Geometry: see drawing. Coordinates: mm, zero at the bounding-box minimum. A direction names the side the tool comes from. Give positions to 0.01 mm unless a question says otherwise; leave off trailing zeros. Write each loop counter-clockwise with the first axis right and the second up, starting at its lowest first coordinate (ties: lowest second). Pieces come first, ordered by that corner, then holes. Notation, with made-up numbers: (61.25, 89) - (104.25, 89) arc R13 ccw to (104.25, 101) - close; hole circle Ø9 at (56, -31.5). An arc over 180 degrees is marked (long way). Use a Markdown table: item, result. Add a question column.
1. Set-up query: the marked faces 1 and 2. Return all of +Z, -Z, +X, -X, +Y, -Y with unobstructed straight access to the full face (end or side cutting, diameter ignored); none if empty.
2. Section query B-B, the plane x = 38.5. Return loops of the section in (y, z).
3. Material intervals for probe 1 along Y at (x, z) = (8.5, 40.5); probe 2 along X at (y, z) = (122.5, 32), sorted ascending.
4. Section query A-A, the plane z = 35. Return loops of the section in (x, y), plus the area to 3 significant figures.
5. Pin query (flat end, axial travel): pin 1 (7.5 mm diameter, centred on x = 35, z = 41.5, fed in from +Y); pin 2 (12 mm diameter, centred on x = 18, z = 12.5, fed in from -Y). Return the tip coordinate at first contact, or that it passes through.
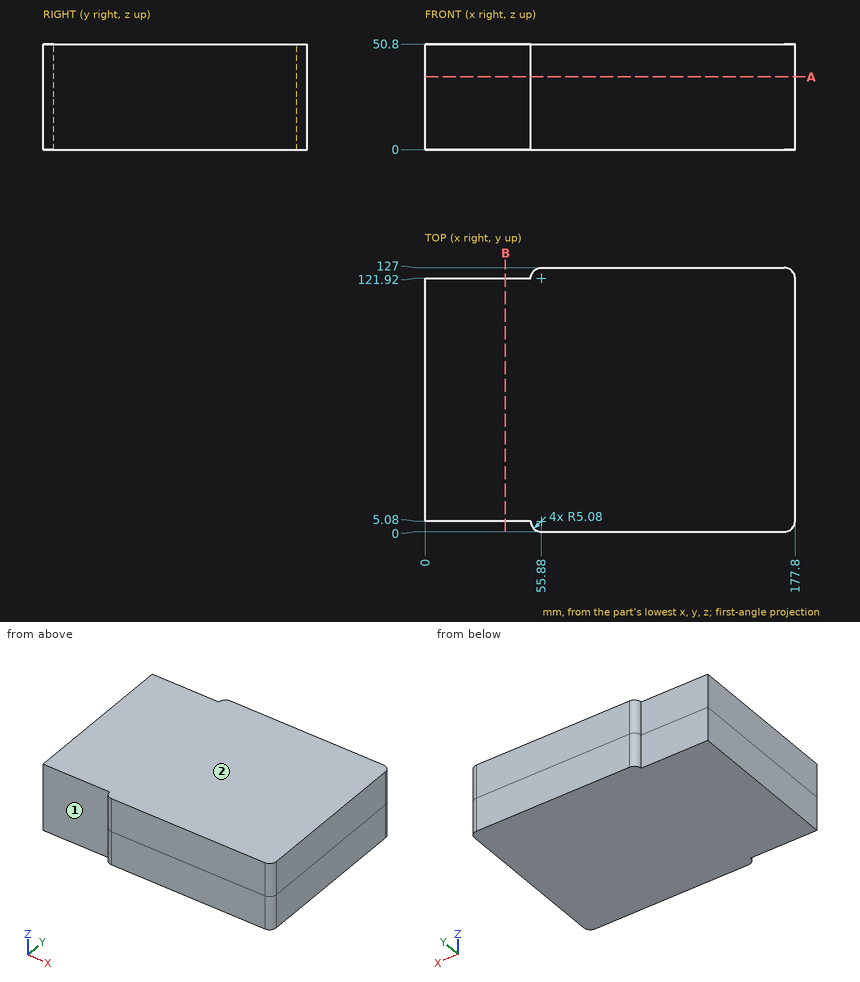
Result sheet:
| question | item | result |
|---|---|---|
| 1 | face 1 | +Z, -Z, -X, -Y |
| 1 | face 2 | +Z, +X, -X, +Y, -Y |
| 2 | outline | (5.08, 0) - (121.92, 0) - (121.92, 50.8) - (5.08, 50.8) - close |
| 3 | probe 1 | y = 5.08 to 121.92 |
| 3 | probe 2 | x = 50.83 to 177.77 |
| 4 | outline | (0, 5.08) - (50.8, 5.08) arc R5.08 ccw to (55.88, 0) - (172.72, 0) arc R5.08 ccw to (177.8, 5.08) - (177.8, 121.92) arc R5.08 ccw to (172.72, 127) - (55.88, 127) arc R5.08 ccw to (50.8, 121.92) - (0, 121.92) - close |
| 4 | area | 22,000 mm² |
| 5 | pin 1 | stops at y = 121.92 |
| 5 | pin 2 | stops at y = 5.08 |
